from build123d import *

# Parameters (mm, degrees)
SKETCH1_R           = 15
SKETCH1_R_2         = 0.9
BOSS_EXTRUDE1_DEPTH = 3
SKETCH2_R           = 7
CUT_EXTRUDE1_DEPTH  = 5.5


with BuildPart() as part:
    # Sketch1 → Boss-Extrude1 (new body)
    with BuildSketch(Plane.XY):
        Circle(SKETCH1_R)
        with Locations((0, -10)):
            Circle(SKETCH1_R_2, mode=Mode.SUBTRACT)
        with Locations((-10, 0)):
            Circle(SKETCH1_R_2, mode=Mode.SUBTRACT)
        with Locations((0, 10)):
            Circle(SKETCH1_R_2, mode=Mode.SUBTRACT)
        with Locations((10, 0)):
            Circle(SKETCH1_R_2, mode=Mode.SUBTRACT)
    extrude(amount=BOSS_EXTRUDE1_DEPTH)

    # Sketch2 → Cut-Extrude1 (cut)
    with BuildSketch(Plane(origin=(0, 0, 0), x_dir=(-1, 0, 0), z_dir=(0, 0, -1))):
        Circle(SKETCH2_R)
    extrude(amount=-CUT_EXTRUDE1_DEPTH, mode=Mode.SUBTRACT)


solid = part.part
Can you work these out from the model? Positions are in its coordinate system, mm. Give positions to 0.01 mm unless a question says otherwise; leave off trailing zeros. Loops run counter-clockwise (first coordinate to the right, second up) from the corner with the lowest first, then second, coordinate; pieces in that order, holes last. Notation, with made-up numbers: (-1.5, 47) -> (11.5, 47) arc R22 cw to (11.5, 85) -> close; hole circle Ø1 at (-22.5, 35). An arc over 180 degrees is marked (long way). Return JSON: item names as keys, results as strings.
Q1. I want a section at A-A, the plane y = 0. List the corners of the cut face in (x, z) for me, then the cut area to 3 significant figures.
Checks:
{"outline": "(-15, 0) -> (-10.9, 0) -> (-10.9, 3) -> (-15, 3) -> close; (-9.1, 0) -> (-7, 0) -> (-7, 3) -> (-9.1, 3) -> close; (7, 0) -> (9.1, 0) -> (9.1, 3) -> (7, 3) -> close; (10.9, 0) -> (15, 0) -> (15, 3) -> (10.9, 3) -> close", "area": "37.2 mm2"}
Q2. We'd pull the mould along X, two halves only. Please class faces 1 (the face through (10.86, 0.27, 1.48)), 2 (the face through (-14.985, 0.66, 1.479)), 3 (the face through (6.5, -3.1, 3)): released by +X, released by -X, zero draft, split by the parting line, or undercut.
Checks:
{"face 1": "undercut", "face 2": "split by the parting line", "face 3": "zero draft"}
Q3. I want a section at D-D, the plane x = -10. List the corners of the cut face in (y, z) for me.
Checks:
{"outline": "(-11.18, 0) -> (-0.9, 0) -> (-0.9, 3) -> (-11.18, 3) -> close; (0.9, 0) -> (11.18, 0) -> (11.18, 3) -> (0.9, 3) -> close"}
Q4. For pin 1 Ø3 at (x, y) = (0, -10) entering from -Z; pin 2 Ø1.5 at (y, z) = (-6.5, 1.5) entering from +X, each with a flat end and sliding along its axis, tell me the tip position at first contact or that it passes through.
Checks:
{"pin 1": "stops at z = 0", "pin 2": "stops at x = 13.85"}
Q5. I need wall thicknesses on probe 1 along Y at (x, z) = (0, 2.25); probe 2 along Y at (x, z) = (-0.75, 0.6); probe 3 along X at (y, z) = (-4.5, 1.7). Which ranges of each line are inside material? Lowest first, please.
Checks:
{"probe 1": "y = -15 to -10.9, -9.1 to -7, 7 to 9.1, 10.9 to 15", "probe 2": "y = -14.98 to -10.5, -9.5 to -6.96, 6.96 to 9.5, 10.5 to 14.98", "probe 3": "x = -14.31 to -5.36, 5.36 to 14.31"}
Q6. I want a section at B-B, the plane z = 1.4. List the corners of the cut face in (x, y) for me, then the cut area to 3 significant figures.
Checks:
{"outline": "circle Ø30 at (0, 0); hole circle Ø1.8 at (-10, 0); hole circle Ø14 at (0, 0); hole circle Ø1.8 at (0, -10); hole circle Ø1.8 at (0, 10); hole circle Ø1.8 at (10, 0)", "area": "543 mm2"}
